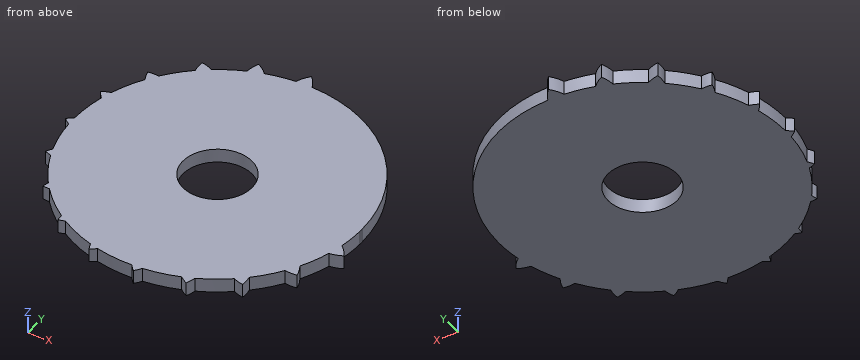
```python
from build123d import *

# Parameters (mm, degrees)
F1_R     = 2.5
F2_DEPTH = 1


with BuildPart() as f2:
    # F1 (on Top) → F2 (new body)
    with BuildSketch(Plane.XY):
        with BuildLine():
            ThreePointArc((10.4010177666, 0.2791052033), (7.3183650566, 7.3959856133), (0.1693586543, 10.4033834852))
            ThreePointArc((0.1693586543, 10.4033834852), (-0.4084890354, 10.3967402104), (-0.9850766389, 10.358025599))
            ThreePointArc((-0.9850766389, 10.358025599), (-2.0168567686, 10.2074168657), (-3.0283814682, 9.9542943486))
            ThreePointArc((-3.0283814682, 9.9542943486), (-3.5459501656, 9.7818867156), (-4.0537711259, 9.5825888962))
            ThreePointArc((-4.0537711259, 9.5825888962), (-5.0373972408, 9.1040485134), (-5.9653480877, 8.5248866554))
            ThreePointArc((-5.9653480877, 8.5248866554), (-6.3706851973, 8.2263868382), (-6.7611105438, 7.9086316458))
            ThreePointArc((-6.7611105438, 7.9086316458), (-7.5960763624, 7.1104637114), (-8.3374242637, 6.2246627975))
            ThreePointArc((-8.3374242637, 6.2246627975), (-8.6009812596, 5.8550996291), (-8.8481688232, 5.4743930047))
            ThreePointArc((-8.8481688232, 5.4743930047), (-9.4287165512, 4.3998152793), (-9.8793415326, 3.2646104174))
            ThreePointArc((-9.8793415326, 3.2646104174), (-9.9979773753, 2.8808885258), (-10.1017152215, 2.4928738192))
            ThreePointArc((-10.1017152215, 2.4928738192), (-10.3320366233, 1.228042959), (-10.4046136849, -0.0555370437))
            ThreePointArc((-10.4046136849, -0.0555370437), (-10.3967402104, -0.4084890354), (-10.3768971195, -0.7609707396))
            ThreePointArc((-10.3768971195, -0.7609707396), (-10.193126284, -2.0878809482), (-9.8403979466, -3.3801832122))
            ThreePointArc((-9.8403979466, -3.3801832122), (-9.7333865621, -3.676990118), (-9.6174251884, -3.9704159783))
            ThreePointArc((-9.6174251884, -3.9704159783), (-9.0097773066, -5.204131357), (-8.2447283135, -6.3469303865))
            ThreePointArc((-8.2447283135, -6.3469303865), (-8.061087037, -6.5785975768), (-7.8709383234, -6.8049540927))
            ThreePointArc((-7.8709383234, -6.8049540927), (-6.8959867768, -7.7913051967), (-5.7985154997, -8.6392296123))
            ThreePointArc((-5.7985154997, -8.6392296123), (-5.549424479, -8.8013043491), (-5.2958064015, -8.9561992414))
            ThreePointArc((-5.2958064015, -8.9561992414), (-4.0708941637, -9.5753272008), (-2.7751475554, -10.0278425566))
            ThreePointArc((-2.7751475554, -10.0278425566), (-2.4655602512, -10.1084164409), (-2.1536422724, -10.1794349184))
            ThreePointArc((-2.1536422724, -10.1794349184), (-0.8330496502, -10.3713595336), (0.5012461634, -10.3926812026))
            ThreePointArc((0.5012461634, -10.3926812026), (0.8600204589, -10.3691578783), (1.2177678025, -10.3332527248))
            ThreePointArc((1.2177678025, -10.3332527248), (2.476254211, -10.105802065), (3.6973306562, -9.725678193))
            ThreePointArc((3.6973306562, -9.725678193), (4.0769602691, -9.5727459623), (4.4502816898, -9.4050020296))
            ThreePointArc((4.4502816898, -9.4050020296), (5.5153513374, -8.8226962954), (6.5053546396, -8.1203098037))
            ThreePointArc((6.5053546396, -8.1203098037), (6.8591715093, -7.823735457), (7.1994838987, -7.5117575764))
            ThreePointArc((7.1994838987, -7.5117575764), (7.983010793, -6.6731258772), (8.6694062261, -5.7533004425))
            ThreePointArc((8.6694062261, -5.7533004425), (8.9411374277, -5.3211964626), (9.1913496147, -4.8762857335))
            ThreePointArc((9.1913496147, -4.8762857335), (9.6500459533, -3.8904605631), (10.0033580362, -2.8621492438))
            ThreePointArc((10.0033580362, -2.8621492438), (10.1409184183, -2.3282705875), (10.2500070535, -1.7878550549))
            ThreePointArc((10.2500070535, -1.7878550549), (10.3660009938, -0.8972701323), (10.4047619048, 0))
            ThreePointArc((10.4047619048, 0), (10.4038258281, 0.1395651578), (10.4010177666, 0.2791052033))
        make_face()
        Circle(F1_R, mode=Mode.SUBTRACT)
        with BuildLine():
            ThreePointArc((-0.9850766389, 10.358025599), (-0.4084890354, 10.3967402104), (0.1693586543, 10.4033834852))
            ThreePointArc((0.1693586543, 10.4033834852), (-0.0915577789, 10.8736948256), (-0.4432176074, 11.280641391))
            ThreePointArc((-0.4432176074, 11.280641391), (-0.7618647264, 10.8473583939), (-0.9850766389, 10.358025599))
        make_face()
        with BuildLine():
            ThreePointArc((-4.0537711259, 9.5825888962), (-3.5459501656, 9.7818867156), (-3.0283814682, 9.9542943486))
            ThreePointArc((-3.0283814682, 9.9542943486), (-3.3994309889, 10.2837794802), (-3.8260663696, 10.5371970223))
            ThreePointArc((-3.8260663696, 10.5371970223), (-3.9851262119, 10.0706763942), (-4.0537711259, 9.5825888962))
        make_face()
        with BuildLine():
            ThreePointArc((10.9249748031, -2.5617942214), (10.6258758179, -2.1413484121), (10.2500070535, -1.7878550549))
            ThreePointArc((10.2500070535, -1.7878550549), (10.1409184183, -2.3282705875), (10.0033580362, -2.8621492438))
            ThreePointArc((10.0033580362, -2.8621492438), (10.4782123863, -2.7550707236), (10.9249748031, -2.5617942214))
        make_face()
        with BuildLine():
            ThreePointArc((-6.7611105438, 7.9086316458), (-6.3706851973, 8.2263868382), (-5.9653480877, 8.5248866554))
            ThreePointArc((-5.9653480877, 8.5248866554), (-6.3783708882, 8.691089302), (-6.8136097843, 8.784781654))
            ThreePointArc((-6.8136097843, 8.784781654), (-6.8244021361, 8.3444870809), (-6.7611105438, 7.9086316458))
        make_face()
        with BuildLine():
            ThreePointArc((9.5380453186, -5.7355619953), (9.4030800104, -5.2904375026), (9.1913496147, -4.8762857335))
            ThreePointArc((9.1913496147, -4.8762857335), (8.9411374277, -5.3211964626), (8.6694062261, -5.7533004425))
            ThreePointArc((8.6694062261, -5.7533004425), (9.1044680071, -5.7807779267), (9.5380453186, -5.7355619953))
        make_face()
        with BuildLine():
            ThreePointArc((-8.8481688232, 5.4743930047), (-8.6009812596, 5.8550996291), (-8.3374242637, 6.2246627975))
            ThreePointArc((-8.3374242637, 6.2246627975), (-8.7265255483, 6.2387786553), (-9.1134062865, 6.1949339122))
            ThreePointArc((-9.1134062865, 6.1949339122), (-9.0073910178, 5.8248704891), (-8.8481688232, 5.4743930047))
        make_face()
        with BuildLine():
            ThreePointArc((7.2382488163, -8.3254097371), (7.2507593771, -7.9170641742), (7.1994838987, -7.5117575764))
            ThreePointArc((7.1994838987, -7.5117575764), (6.8591715093, -7.823735457), (6.5053546396, -8.1203098037))
            ThreePointArc((6.5053546396, -8.1203098037), (6.8642964884, -8.2496786303), (7.2382488163, -8.3254097371))
        make_face()
        with BuildLine():
            ThreePointArc((-10.1017152215, 2.4928738192), (-9.9979773753, 2.8808885258), (-9.8793415326, 3.2646104174))
            ThreePointArc((-9.8793415326, 3.2646104174), (-10.1976364828, 3.162779516), (-10.500335771, 3.0211661383))
            ThreePointArc((-10.500335771, 3.0211661383), (-10.3178144144, 2.7443519774), (-10.1017152215, 2.4928738192))
        make_face()
        with BuildLine():
            ThreePointArc((4.2507054017, -10.0778251054), (4.373179067, -9.7481426651), (4.4502816898, -9.4050020296))
            ThreePointArc((4.4502816898, -9.4050020296), (4.0769602691, -9.5727459623), (3.6973306562, -9.725678193))
            ThreePointArc((3.6973306562, -9.725678193), (3.9629273196, -9.919179939), (4.2507054017, -10.0778251054))
        make_face()
        with BuildLine():
            ThreePointArc((-10.3768971195, -0.7609707396), (-10.3967402104, -0.4084890354), (-10.4046136849, -0.0555370437))
            ThreePointArc((-10.4046136849, -0.0555370437), (-10.6317595983, -0.2288157362), (-10.8386359166, -0.425851165))
            ThreePointArc((-10.8386359166, -0.425851165), (-10.6169381073, -0.6060478704), (-10.3768971195, -0.7609707396))
        make_face()
        with BuildLine():
            ThreePointArc((0.8678566395, -10.8212694742), (1.0568743578, -10.5873437424), (1.2177678025, -10.3332527248))
            ThreePointArc((1.2177678025, -10.3332527248), (0.8600204589, -10.3691578783), (0.5012461634, -10.3926812026))
            ThreePointArc((0.5012461634, -10.3926812026), (0.6729569444, -10.6168931305), (0.8678566395, -10.8212694742))
        make_face()
        with BuildLine():
            ThreePointArc((-9.6174251884, -3.9704159783), (-9.7333865621, -3.676990118), (-9.8403979466, -3.3801832122))
            ThreePointArc((-9.8403979466, -3.3801832122), (-9.978035392, -3.5883525406), (-10.0951915478, -3.8086999272))
            ThreePointArc((-10.0951915478, -3.8086999272), (-9.8602185944, -3.901110143), (-9.6174251884, -3.9704159783))
        make_face()
        with BuildLine():
            ThreePointArc((-2.5791606638, -10.4829693286), (-2.3587946678, -10.341865934), (-2.1536422724, -10.1794349184))
            ThreePointArc((-2.1536422724, -10.1794349184), (-2.4655602512, -10.1084164409), (-2.7751475554, -10.0278425566))
            ThreePointArc((-2.7751475554, -10.0278425566), (-2.6879646474, -10.2600611812), (-2.5791606638, -10.4829693286))
        make_face()
        with BuildLine():
            ThreePointArc((-7.8709383234, -6.8049540927), (-8.061087037, -6.5785975768), (-8.2447283135, -6.3469303865))
            ThreePointArc((-8.2447283135, -6.3469303865), (-8.3036538881, -6.5694261546), (-8.3427761795, -6.7962433419))
            ThreePointArc((-8.3427761795, -6.7962433419), (-8.1070542554, -6.8112698876), (-7.8709383234, -6.8049540927))
        make_face()
        with BuildLine():
            ThreePointArc((-5.7529284377, -9.0960398441), (-5.5211636058, -9.036592423), (-5.2958064015, -8.9561992414))
            ThreePointArc((-5.2958064015, -8.9561992414), (-5.549424479, -8.8013043491), (-5.7985154997, -8.6392296123))
            ThreePointArc((-5.7985154997, -8.6392296123), (-5.7857710928, -8.8686375736), (-5.7529284377, -9.0960398441))
        make_face()
    extrude(amount=F2_DEPTH)


solid = f2.part
```
Read the model definition and answer for the solid it produces. Units are mm, in the model's axes. Give positions to 0.01 mm unless a question says otherwise; leave off trailing zeros. Write each loop counter-clockwise with the first axis right and the second up, starting at its lowest first coordinate (ties: lowest second). Pieces come first, ordered by that corner, then holes. Notation, with made-up numbers: M -15.5,-5 L 17.5,-5 A28 ccw 17.5,28 Z; hole C 36,-35.75 d9. An arc over 180 degrees is marked long. Put each result on its own line as item: value. Start each with the question number.
1. Consider line 1 along Y through (x, z) = (0, 0.4); line 2 along X through (y, z) = (1.5, 0.35); line 3 along Y through (x, z) = (-0.75, 0.3). Determine where each line is inside the solid, lowest interval first.
2. This flat-tipped pin is pushed along its axis until it touches: pin 1 Ø1 at (x, y) = (7, -7) entering from -Z. Where does it stop, or does it pass through?
3. The part is cut by section A-A, the plane x = 8.25. Give the vertices of the cut face in (y, z), and give its area (3 significant figures).
Final values:
1. line 1: y = -10.4 to -2.5, 2.5 to 10.73
1. line 2: x = -10.3 to -2, 2 to 10.3
1. line 3: y = -10.38 to -2.38, 2.38 to 10.87
2. pin 1: stops at z = 0
3. outline: M -6.34,0 L 6.34,0 L 6.34,1 L -6.34,1 Z
3. area: 12.7 mm²
